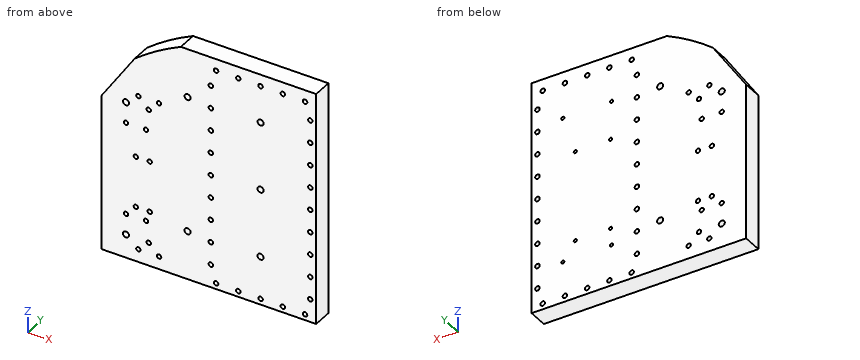
Autodesk Inventor part; units mm, degrees
ref_plane "YZ Plane" through (0, 0, 0) normal (1, 0, 0) x (0, 1, 0)
ref_plane "XZ Plane" through (0, 0, 0) normal (0, 1, 0) x (-1, 0, 0)
ref_plane "XY Plane" through (0, 0, 0) normal (0, 0, 1) x (1, 0, 0)
sketch "Sketch1" plane through (0, 0, 0) normal (0, 1, 0) x (-1, 0, 0)
  line L0 (69.85, 76.2) -> (-69.85, 76.2)
  line L1 (-69.85, 76.2) -> (-69.85, -76.2)
  line L2 (-69.85, -76.2) -> (69.85, -76.2)
  line L3 (69.85, -76.2) -> (69.85, 76.2)
  point P0 (0, 0)
  dimension "d0" = 152.4
  dimension "d1" = 139.7
  dimension "d2" = 69.85
  dimension "d3" = 76.2
extrude "Extrusion1" add sketch "Sketch1" along normal blind 12.7
fillet "Fillet1" [suppressed]
sketch "Sketch7" plane through (0, 12.7, 0) normal (0, 1, 0) x (1, 0, 0)
  arc A0 (-69.85, -37.0366) -> (-18.2851, -76.2) centre (46.0045, 61.976) ccw
  line L0 (69.85, 76.2) -> (-69.85, 76.2)
  line L1 (69.85, -76.2) -> (69.85, 76.2)
  line L2 (-69.85, 76.2) -> (-69.85, -76.2)
  line L3 (-69.85, -76.2) -> (69.85, -76.2)
  line L4 (-69.85, 76.2) -> (-69.85, -76.2)
  arc A1 (-18.2851, -76.2) -> (-69.85, -37.0366) centre (46.0045, 61.976) ccw
  point P0 (0, 0)
  point P1 (76.2, -60.325)
  point P2 (73.025, -60.325)
  point P3 (73.025, 63.5)
  point P4 (73.025, 60.325)
  point P5 (-73.025, 63.5)
  point P6 (76.2, 60.325)
  point P7 (73.025, -63.5)
  point P8 (-76.2, 60.325)
  point P9 (-80.9955, -22.2663)
  dimension "d46" = 304.8
  dimension "d47" = 14.224
  dimension "d48" = 23.8455
sketch "Sketch8" plane through (0, 12.7, 0) normal (0, 1, 0) x (1, 0, 0)
  circle A0 centre (-47.526, 7.0319) radius 1.4224
  circle A1 centre (-47.526, 7.0319) radius 1.4224
  circle A2 centre (-38.506, 7.0319) radius 1.4224
  line L0 (-33.996, 3.9778) -> (-52.036, 3.9778)
  line L1 (-33.996, 10.086) -> (-33.996, 3.9778)
  line L2 (-33.996, 10.086) -> (-52.036, 10.086)
  line L3 (-52.036, 3.9778) -> (-52.036, 10.086)
  circle A3 centre (-47.526, 40.2937) radius 1.4224
  circle A4 centre (-38.506, 40.2937) radius 1.4224
  line L4 (-33.996, 37.2396) -> (-52.036, 37.2396)
  line L5 (-33.996, 43.3478) -> (-33.996, 37.2396)
  line L6 (-33.996, 43.3478) -> (-52.036, 43.3478)
  line L7 (-52.036, 37.2396) -> (-52.036, 43.3478)
  circle A5 centre (2.54, -39.6875) radius 3.175 construction
  circle A6 centre (2.54, 12.7127) radius 3.175 construction
  circle A7 centre (2.54, 65.1129) radius 3.175 construction
  circle A8 centre (68.58, 65.1129) radius 3.175 construction
  circle A9 centre (68.58, 12.7127) radius 3.175 construction
  circle A10 centre (68.58, -39.6875) radius 3.175 construction
  circle A11 centre (-32.4275, -33.782) radius 1.4224
  circle A12 centre (-39.1585, -27.051) radius 1.4224
  circle A13 centre (-45.8895, -33.782) radius 1.4224
  circle A14 centre (-45.8895, 67.818) radius 1.4224
  circle A15 centre (-39.1585, 61.087) radius 1.4224
  circle A16 centre (-32.4275, 67.818) radius 1.4224
extrude "Extrusion9" cut sketch "Sketch8" against normal through all contours A0 | A2 | A3 | A4 | A11 | A12 | A13 | A14 | A15 | A16
extrude "Extrusion11" cut sketch "Sketch7" against normal through all contours A0 L3 L2
sketch "Sketch10" plane through (0, 12.7, 0) normal (0, 1, 0) x (1, 0, 0)
  circle A0 centre (62.611, 72.39) radius 1.4732
  arc A1 (-69.85, -37.0366) -> (-18.2851, -76.2) centre (46.0045, 61.976) ccw
  line L0 (-18.2851, -76.2) -> (69.85, -76.2)
  line L1 (69.85, -76.2) -> (69.85, 76.2)
  line L2 (69.85, 76.2) -> (-69.85, 76.2)
  line L3 (-69.85, 76.2) -> (-69.85, -37.0366)
  circle A2 centre (-47.526, 40.2937) radius 1.4224
  circle A3 centre (-47.526, 7.0319) radius 1.4224
  circle A4 centre (-38.506, 7.0319) radius 1.4224
  circle A5 centre (-38.506, 40.2937) radius 1.4224
  circle A6 centre (33.655, 72.39) radius 1.4732
  circle A7 centre (48.133, 72.39) radius 1.4732
  circle A8 centre (19.177, 72.39) radius 1.4732
  circle A9 centre (4.699, 72.39) radius 1.4732
  circle A10 centre (62.611, -68.58) radius 1.4732
  circle A11 centre (48.133, -68.58) radius 1.4732
  circle A12 centre (33.655, -68.58) radius 1.4732
  circle A13 centre (19.177, -68.58) radius 1.4732
  circle A14 centre (4.699, -68.58) radius 1.4732
  point P0 (0, 0)
extrude "Extrusion13" cut sketch "Sketch10" against normal through all contours A0 | A6 | A7 | A8 | A9 | A10 | A11 | A12 | A13 | A14
sketch "Sketch11" plane through (0, 12.7, 0) normal (0, 1, 0) x (1, 0, 0)
  circle A0 centre (19.177, 72.39) radius 1.4732
  circle A1 centre (48.133, 72.39) radius 1.4732
  circle A2 centre (62.611, -68.58) radius 1.4732
  circle A3 centre (33.655, -68.58) radius 1.4732
  circle A4 centre (4.699, -68.58) radius 1.4732
  circle A5 centre (1.27, -42.545) radius 1.4732
  circle A6 centre (1.27, -12.9117) radius 1.4732
  circle A7 centre (1.27, 16.7217) radius 1.4732
  circle A8 centre (1.27, 46.355) radius 1.4732
  circle A9 centre (66.04, 61.1717) radius 1.4732
  circle A10 centre (66.04, 31.5383) radius 1.4732
  circle A11 centre (66.04, 1.905) radius 1.4732
  circle A12 centre (66.04, -27.7283) radius 1.4732
  circle A13 centre (66.04, -57.3617) radius 1.4732
  circle A14 centre (66.04, -42.545) radius 1.4732
  circle A15 centre (66.04, -12.9117) radius 1.4732
  circle A16 centre (66.04, 16.7217) radius 1.4732
  circle A17 centre (66.04, 46.355) radius 1.4732
  circle A18 centre (1.27, 61.1717) radius 1.4732
  circle A19 centre (1.27, 31.5383) radius 1.4732
  circle A20 centre (1.27, 1.905) radius 1.4732
  circle A21 centre (1.27, -27.7283) radius 1.4732
  circle A22 centre (1.27, -57.3617) radius 1.4732
  circle A23 centre (19.177, -68.58) radius 1.4732
  circle A24 centre (48.133, -68.58) radius 1.4732
  circle A25 centre (62.611, 72.39) radius 1.4732
  circle A26 centre (33.655, 72.39) radius 1.4732
  circle A27 centre (4.699, 72.39) radius 1.4732
  line L0 (0.635, -72.39) -> (66.675, -72.39)
  line L1 (69.85, -69.215) -> (69.85, 73.025)
  line L2 (66.675, 76.2) -> (0.635, 76.2)
  line L3 (-2.54, 73.025) -> (-2.54, -69.215)
  arc A28 (59.055, 62.23) -> (55.88, 65.405) centre (55.88, 62.23) ccw
  line L4 (59.055, -58.42) -> (59.055, 62.23)
  arc A29 (55.88, -61.595) -> (59.055, -58.42) centre (55.88, -58.42) ccw
  line L5 (11.43, -61.595) -> (55.88, -61.595)
  arc A30 (8.255, -58.42) -> (11.43, -61.595) centre (11.43, -58.42) ccw
  line L6 (8.255, 62.23) -> (8.255, -58.42)
  arc A31 (11.43, 65.405) -> (8.255, 62.23) centre (11.43, 62.23) ccw
  line L7 (55.88, 65.405) -> (11.43, 65.405)
  arc A32 (69.85, 73.025) -> (66.675, 76.2) centre (66.675, 73.025) ccw
  arc A33 (0.635, 76.2) -> (-2.54, 73.025) centre (0.635, 73.025) ccw
  arc A34 (-2.54, -69.215) -> (0.635, -72.39) centre (0.635, -69.215) ccw
  arc A35 (66.675, -72.39) -> (69.85, -69.215) centre (66.675, -69.215) ccw
  point P0 (0, 0)
  point P1 (52.705, -61.595)
extrude "Extrusion14" cut sketch "Sketch11" against normal through all contours A5 | A6 | A7 | A8 | A9 | A10 | A11 | A12 | A13 | A14 | A15 | A16 | A17 | A18 | A19 | A20 | A21 | A22 | A25
sketch "Sketch14" plane through (0, 0, 0) normal (0, -1, 0) x (1, 0, 0)
  line L0 (69.85, -76.2) -> (-69.85, -76.2)
  line L1 (-18.2851, 76.2) -> (69.85, 76.2)
  circle A0 centre (4.699, -72.39) radius 1.4732
  circle A1 centre (-32.4275, -67.818) radius 1.4224
  point P0 (0, 0)
  point P1 (-13.8643, 44.45)
  point P2 (-13.8643, -44.45)
  dimension "d79" = 44.45
  dimension "d80" = 152.4
  dimension "d81" = 44.45
  dimension "d82" = 37.1265
  dimension "d83" = 18.5633
  dimension "d84" = 18.5633
hole "Hole2" at (-13.8643, 0, 44.45) at (-13.8643, 0, -44.45) direction (0, 1, 0) diameter 3.9624 end through all
sketch "Sketch15" plane through (0, 0, 0) normal (0, -1, 0) x (1, 0, 0)
  circle A0 centre (-13.8643, 44.45) radius 1.9812
  circle A1 centre (-13.8643, -44.45) radius 1.9812
  circle A2 centre (66.04, -31.5383) radius 1.4732
  circle A3 centre (1.27, -31.5383) radius 1.4732
  circle A4 centre (1.27, 42.545) radius 1.4732
  point P0 (0, 0)
  point P1 (33.655, -44.45)
  point P2 (33.655, 44.45)
  point P3 (33.655, 0)
  dimension "d92" = 44.45
  dimension "d93" = 44.45
  dimension "d94" = 44.45
  dimension "d95" = 44.45
  dimension "d96" = 64.77
  dimension "d97" = 32.385
  dimension "d98" = 32.385
  dimension "d222" = 32.385
  dimension "d223" = 44.45
hole "Hole3" at (33.655, 0, -44.45) at (33.655, 0, 44.45) at (33.655, 0, 0) direction (0, 1, 0) diameter 3.9624 depth 9.525
thread "Thread3"
thread "Thread4"
thread "Thread5"
thread "Thread6"
thread "Thread7"
thread "Thread8"
thread "Thread9"
thread "Thread10"
thread "Thread11"
thread "Thread12"
thread "Thread13"
thread "Thread14"
thread "Thread15"
thread "Thread16"
thread "Thread17"
thread "Thread18"
thread "Thread19"
thread "Thread20"
thread "Thread21"
thread "Thread22"
thread "Thread23"
thread "Thread24"
thread "Thread25"
thread "Thread26"
thread "Thread27"
thread "Thread28"
thread "Thread29"
thread "Thread30"
thread "Thread31"
thread "Thread32"
thread "Thread33"
thread "Thread34"
thread "Thread35"
thread "Thread36"
thread "Thread37"
thread "Thread38"
thread "Thread39"
thread "Thread40"
thread "Thread41"
sketch "Sketch17" plane through (0, 12.7, 0) normal (0, 1, 0) x (1, 0, 0)
  line L0 (-48.26, -57.7736) -> (-69.85, -25.6538)
  line L1 (-69.85, 76.2) -> (-69.85, -37.0366)
  line L2 (-69.85, -25.6538) -> (-69.85, -37.0366)
  arc A0 (-69.85, -37.0366) -> (-18.2851, -76.2) centre (46.0045, 61.976) ccw
  arc A1 (-69.85, -37.0366) -> (-48.26, -57.7736) centre (46.0045, 61.976) ccw
  point P0 (0, 0)
  dimension "d200" = 6.35
  dimension "d203" = 21.59
extrude "Extrusion16" cut sketch "Sketch17" against normal through all
thread "Thread46"
thread "Thread47"
thread "Thread48"
sketch "Sketch19" plane through (0, 12.7, 0) normal (0, 1, 0) x (1, 0, 0)
  circle A0 centre (49.53, 49.53) radius 1.025
  line L0 (-18.2851, -76.2) -> (69.85, -76.2)
  line L1 (69.85, -76.2) -> (69.85, 76.2)
  line L2 (69.85, 76.2) -> (-69.85, 76.2)
  circle A1 centre (49.53, -45.72) radius 1.025
  circle A2 centre (17.78, 49.53) radius 1.025
  circle A3 centre (17.78, -45.72) radius 1.025
  circle A4 centre (18.415, -20.745) radius 1.0287
  circle A5 centre (18.415, 38.255) radius 1.0287
  circle A6 centre (41.415, -20.745) radius 1.0287
  circle A7 centre (41.415, 38.255) radius 1.0287
  point P0 (0, 0)
  point P1 (-28.9602, -57.9611)
  point P2 (18.415, 8.255)
  dimension "d239" = 2.05
  dimension "d241" = 20.32
  dimension "d242" = 26.67
  dimension "d245" = 95.25
  dimension "d248" = 31.75
  dimension "d251" = 31.115
  dimension "d252" = 53.975
  dimension "d253" = 2.0574
  dimension "d254" = 29
  dimension "d257" = 59
  dimension "d260" = 23
sketch "Sketch18" plane through (0, 12.7, 0) normal (0, 1, 0) x (1, 0, 0)
  circle A0 centre (-47.6269, -14.097) radius 2.794
  circle A1 centre (-47.6269, 48.133) radius 2.794
  point P0 (0, 0)
  point P1 (-53.9769, 60.833)
  point P2 (-53.9769, -26.797)
  dimension "d211" = 12.7
  dimension "d212" = 12.7
  dimension "d213" = 6.35
  dimension "d214" = 6.35
hole "Hole4" at (-53.9769, 12.7, -60.833) at (-53.9769, 12.7, 26.797) direction (0, -1, 0) diameter 3.9624 depth 12.7
sketch "Sketch21" plane through (0, 12.7, 0) normal (0, 1, 0) x (1, 0, 0)
  line L0 (69.85, 76.2) -> (-69.85, 76.2)
  line L1 (-69.85, 76.2) -> (-69.85, -25.6538)
  point P0 (0, 0)
  point P1 (-53.9242, -13.1826)
  point P2 (-40.9194, -13.1826)
  point P3 (-40.9194, 47.1932)
  point P4 (-53.9242, 47.1932)
  dimension "d224" = 29.0068
  dimension "d225" = 15.9258
  dimension "d226" = 28.9306
  dimension "d227" = 29.0068
  dimension "d228" = 15.9258
  dimension "d229" = 89.3826
  dimension "d230" = 89.3826
  dimension "d231" = 28.9306
hole "Hole5" at (-53.9242, 12.7, 13.1826) at (-40.9194, 12.7, 13.1826) at (-53.9242, 12.7, -47.1932) at (-40.9194, 12.7, -47.1932) direction (0, -1, 0) diameter 2.8448 end through all
extrude "Extrusion17" cut sketch "Sketch19" against normal blind 5.08
properties part number "Base Plate Mk 2" material "Aluminum 6061"
Design review of the part built by this model. Coordinates are the model's own, in mm. Round coordinates to 2 decimals unless told otherwise and drop trailing zeros. Write each loop counter-clockwise with the first axis right and the second up, starting at its lowest first coordinate (ties: lowest second). Pieces come first, ordered by that corner, then holes.
Item 1: We need section A-A on y = 3.5. State how many separate pieces and enclosed holes the cut face has, and give its area (3 significant figures).
Item 2: For probe 1 along X at (y, z) = (7.75, -17); probe 2 along X at (y, z) = (10.55, -49.53) (3 decimals); probe 3 along X at (y, z) = (3.5, 68), list the stretches that pass through material, from the lowest coordinate up.
Item 3: We need section B-B on z = 39. Write out the cut boundary in (x, y).
Item 4: Clearance check with flat-ended pins moving along their axes: pin 1 Ø1.5 at (y, z) = (7, 58) entering from -X; pin 2 Ø3 at (y, z) = (11, 27.5) entering from -X; pin 3 Ø0.6 at (x, z) = (17.5, -50) entering from +Y. State where each tip first meets the part, or that it passes through.
Item 5: We need section C-C on x = -60. Write out the cut boundary in (y, z), and give its area (3 significant figures).
Returned:
1. separate pieces: 1
1. enclosed holes: 49
1. area: 19,900 mm2
2. probe 1: x = -69.85 to -0.18, 2.72 to 64.59, 67.49 to 69.85
2. probe 2: x = -69.85 to 16.755, 18.805 to 48.505, 50.555 to 69.85
2. probe 3: x = -33.57 to 3.34, 6.05 to 17.82, 20.53 to 32.3, 35.01 to 46.78, 49.49 to 61.26, 63.97 to 69.85
3. outline: (-60.88, 0) - (69.85, 0) - (69.85, 12.7) - (-60.88, 12.7) - close
4. pin 1: stops at x = -48.61
4. pin 2: stops at x = -69.62
4. pin 3: stops at y = 7.62
5. outline: (0, -76.2) - (12.7, -76.2) - (12.7, 40.31) - (0, 40.31) - close
5. area: 1,480 mm2
